```python
from build123d import *

# Parameters (mm, degrees)
BOSS_EXTRUDE1_DEPTH = 5
SKETCH2_W           = 33
SKETCH2_H           = 20
SKETCH2_W_2         = 10
SKETCH2_H_2         = 10
CUT_EXTRUDE1_DEPTH  = 5
CUT_EXTRUDE2_DEPTH  = 10
SKETCH4_R           = 3
CUT_EXTRUDE3_DEPTH  = 10


with BuildPart() as part:
    # Sketch1 → Boss-Extrude1 (new body)
    with BuildSketch(Plane.XY):
        Polygon((26.5, -31), (26.5, -36), (6.5, -36), (6.5, -31), (-41.5, -31), (-41.5, 31), (41.5, 31), (41.5, -31), align=None)
    extrude(amount=BOSS_EXTRUDE1_DEPTH)

    # Sketch2 → Cut-Extrude1 (cut)
    with BuildSketch(Plane(origin=(0, 0, 0), x_dir=(-1, 0, 0), z_dir=(0, 0, -1))):
        with Locations((25, -21)):
            Rectangle(SKETCH2_W, SKETCH2_H)
        with Locations((-36.5, 26)):
            Rectangle(SKETCH2_W_2, SKETCH2_H_2)
    extrude(amount=-CUT_EXTRUDE1_DEPTH, mode=Mode.SUBTRACT)

    # Sketch3 → Cut-Extrude2 (cut)
    with BuildSketch(Plane(origin=(0, 0, 0), x_dir=(-1, 0, 0), z_dir=(0, 0, -1))):
        Polygon((31.5, 22.6), (31.5, 12.6), (27.1, 12.6), (27.1, 22.6), (25.6, 22.6), (25.6, 26), (27.1, 26), (27.1, 31), (31.5, 31), (31.5, 26), (33, 26), (33, 22.6), align=None)
        Polygon((-17.1, 22.6), (-17.1, 12.6), (-21.5, 12.6), (-21.5, 22.6), (-23, 22.6), (-23, 26), (-21.5, 26), (-21.5, 31), (-17.1, 31), (-17.1, 26), (-15.6, 26), (-15.6, 22.6), align=None)
    extrude(amount=-CUT_EXTRUDE2_DEPTH, mode=Mode.SUBTRACT)

    # Sketch4 → Cut-Extrude3 (cut)
    with BuildSketch(Plane(origin=(0, 0, 0), x_dir=(-1, 0, 0), z_dir=(0, 0, -1))):
        with Locations((29.5, 8)):
            Circle(SKETCH4_R)
        with Locations((-19.5, 8)):
            Circle(SKETCH4_R)
    extrude(amount=-CUT_EXTRUDE3_DEPTH, mode=Mode.SUBTRACT)


solid = part.part
```
Read the model definition and answer for the solid it produces. Units are mm, in the model's axes. A direction names the side the tool comes from. Round coordinates to 2 decimals unless told otherwise and drop trailing zeros. Write each loop counter-clockwise with the first axis right and the second up, starting at its lowest first coordinate (ties: lowest second). Pieces come first, ordered by that corner, then holes. Notation, with made-up numbers: (1, 89.25) -> (56, 89.25) arc R25 ccw to (56, 106.25) -> close; hole circle Ø9 at (67, -12). An arc over 180 degrees is marked (long way). Answer in a Markdown table with one row per item. Add a question column.
1) Find section B-B, the plane y = 8. Determine the outline of the cut face in (x, z).
2) Given P1, Ø2.5, axis at x = 0.5, z = 3, coming from the -Y side; P2, Ø1, axis at x = 33, y = 22.5, coming from the -Z side; P3, Ø1.3, axis at x = 19, z = 2.5, coming from the +Y side; P4, Ø2.5, axis at x = 37, z = 3, coming from the +Y side, each flat-ended and moving along its own axis, determine where each tip first touches the part or whether it passes through.
3) Find section D-D, the plane z = 1.6. State how many separate pieces and enclosed holes the cut face has, and give its area (3 significant figures).
4) Determine the mould class of faces 5 (the face through (-8.5, -21, 2)), 6 (the face through (34, -31, 2)), 7 (the face through (22.5, 8.1, 2.5)) for opening direction Y: pulls with the +Y half, pulls with the -Y half, needs draft (parallel to the pull), parting line crosses it, or undercut.
5) Find section A-A, the plane x = 19.5. Determine the outline of the cut face in (y, z), and give its area (3 significant figures).
6) Find section C-C, the plane y = 20. Determine the outline of the cut face in (x, z), and give its area (3 significant figures).
7) Which of the six approach directions +Z, -Z, +X, -X, +Y, -Y give full straight-line access (tool end or side, diameter ignored) to faces 1 (the face through (31.5, 26, 2)), 2 (the face through (-27.1, 18, 2)), 3 (the face through (1, 5, 5)), 4 (the face through (23, 24, 2))?
8) Consider line 1 (X direction, y = 17, z = 1.35); line 2 (X direction, y = 25.5, z = 0.75); line 3 (Y direction, x = -22, z = 4). Determine where each line is inside the solid, lowest interval first.
Findings below:
| question | item | result |
|---|---|---|
| 1 | outline | (-41.5, 0) -> (-32.5, 0) -> (-32.5, 5) -> (-41.5, 5) -> close; (-26.5, 0) -> (16.5, 0) -> (16.5, 5) -> (-26.5, 5) -> close; (22.5, 0) -> (41.5, 0) -> (41.5, 5) -> (22.5, 5) -> close |
| 2 | P1 | y = -31 |
| 2 | P2 | through |
| 2 | P3 | y = 12.6 |
| 2 | P4 | y = 21 |
| 3 | separate pieces | 1 |
| 3 | enclosed holes | 2 |
| 3 | area | 4,250 mm² |
| 4 | face 5 | needs draft |
| 4 | face 6 | pulls with the -Y half |
| 4 | face 7 | undercut |
| 5 | outline | (-36, 0) -> (5, 0) -> (5, 5) -> (-36, 5) -> close; (11, 0) -> (12.6, 0) -> (12.6, 5) -> (11, 5) -> close |
| 5 | area | 213 mm² |
| 6 | outline | (-41.5, 0) -> (-31.5, 0) -> (-31.5, 5) -> (-41.5, 5) -> close; (-27.1, 0) -> (17.1, 0) -> (17.1, 5) -> (-27.1, 5) -> close; (21.5, 0) -> (41.5, 0) -> (41.5, 5) -> (21.5, 5) -> close |
| 6 | area | 371 mm² |
| 7 | face 1 | +Z, -Z, +X, +Y |
| 7 | face 2 | +Z, -Z, +Y |
| 7 | face 3 | +Z, +X, -X, +Y, -Y |
| 7 | face 4 | +Z, -Z |
| 8 | line 1 | -41.5 to -31.5, -27.1 to 17.1, 21.5 to 41.5 |
| 8 | line 2 | -41.5 to -33, -25.6 to 15.6, 23 to 31.5 |
| 8 | line 3 | -11 to 31 |
